Model file for the job. Use its own axes, mm. A direction names the side the tool comes from. Give positions to 0.01 mm unless a question says otherwise; leave off trailing zeros. Write each loop counter-clockwise with the first axis right and the second up, starting at its lowest first coordinate (ties: lowest second). Pieces come first, ordered by that corner, then holes. Notation, with made-up numbers: M 36,49 L 83,49 A28 cw 83,74 Z; hole C 0.5,-10.5 d2. An arc over 180 degrees is marked long. Answer as a JSON object with one key per item and string values. Group by question number.
```python
from build123d import *

# Parameters (mm, degrees)
F0_R     = 1
F0_W     = 2
F0_H     = 3
F0_R_2   = 12.5
F1_DEPTH = 2
F2_DEPTH = 2


with BuildPart() as f1:
    # F0 (on Top) → F1 (new body)
    with BuildSketch(Plane.XY):
        with BuildLine():
            Line((10, 16), (-10, 16))
            ThreePointArc((-10, 16), (-14.2426406871, 14.2426406871), (-16, 10))
            Line((-16, 10), (-16, -10))
            ThreePointArc((-16, -10), (-14.2426406871, -14.2426406871), (-10, -16))
            Line((-10, -16), (10, -16))
            ThreePointArc((10, -16), (14.2426406871, -14.2426406871), (16, -10))
            Line((16, -10), (16, 10))
            ThreePointArc((16, 10), (14.2426406871, 14.2426406871), (10, 16))
        make_face()
        with Locations((-12, -12)):
            Circle(F0_R, mode=Mode.SUBTRACT)
        with Locations((-13.5, -7.8047601065)):
            Rectangle(F0_W, F0_H, mode=Mode.SUBTRACT)
        with Locations((12, -12)):
            Circle(F0_R, mode=Mode.SUBTRACT)
        with Locations((13.5, -7.8047601065)):
            Rectangle(F0_W, F0_H, mode=Mode.SUBTRACT)
        with Locations((-13.5, 7.8047601065)):
            Rectangle(F0_W, F0_H, mode=Mode.SUBTRACT)
        with Locations((-12, 12)):
            Circle(F0_R, mode=Mode.SUBTRACT)
        Circle(F0_R_2, mode=Mode.SUBTRACT)
        with Locations((13.5, 7.8047601065)):
            Rectangle(F0_W, F0_H, mode=Mode.SUBTRACT)
        with Locations((12, 12)):
            Circle(F0_R, mode=Mode.SUBTRACT)
    extrude(amount=F1_DEPTH)

    # F0 (on Top) → F2 (join)
    with BuildSketch(Plane.XY):
        with BuildLine():
            Line((10, 16), (-10, 16))
            ThreePointArc((-10, 16), (-14.2426406871, 14.2426406871), (-16, 10))
            Line((-16, 10), (-16, -10))
            ThreePointArc((-16, -10), (-14.2426406871, -14.2426406871), (-10, -16))
            Line((-10, -16), (10, -16))
            ThreePointArc((10, -16), (14.2426406871, -14.2426406871), (16, -10))
            Line((16, -10), (16, 10))
            ThreePointArc((16, 10), (14.2426406871, 14.2426406871), (10, 16))
        make_face()
        with Locations((-12, -12)):
            Circle(F0_R, mode=Mode.SUBTRACT)
        with Locations((-13.5, -7.8047601065)):
            Rectangle(F0_W, F0_H, mode=Mode.SUBTRACT)
        with Locations((12, -12)):
            Circle(F0_R, mode=Mode.SUBTRACT)
        with Locations((13.5, -7.8047601065)):
            Rectangle(F0_W, F0_H, mode=Mode.SUBTRACT)
        with Locations((-13.5, 7.8047601065)):
            Rectangle(F0_W, F0_H, mode=Mode.SUBTRACT)
        with Locations((-12, 12)):
            Circle(F0_R, mode=Mode.SUBTRACT)
        Circle(F0_R_2, mode=Mode.SUBTRACT)
        with Locations((13.5, 7.8047601065)):
            Rectangle(F0_W, F0_H, mode=Mode.SUBTRACT)
        with Locations((12, 12)):
            Circle(F0_R, mode=Mode.SUBTRACT)
    extrude(amount=F2_DEPTH)


solid = f1.part
```
Q1. Drop flat-ended pins along their axis: P1, Ø0.6, axis at x = 13, z = 0.5, coming from the -Y side; P2, Ø0.6, axis at x = 14, z = 1, coming from the -Y side; P3, Ø1, axis at x = -14, z = 0.5, coming from the +Y side. Give the stop position or say it passes through.
Q2. Wall check: L1, parallel to X at y = 6.5, z = 0.6; L2, parallel to X at y = -8.5, z = 1.2; L3, parallel to Y at x = 8.5, z = 0.3. Give the ranges that are in metal, low to high.
Q3. Slice it at A-A, the plane x = 0. Write the cut outline in (y, z).
Q4. Slice it at B-B, the plane z = 1.45. Count the separate pieces of the cut face and the enclosed holes in it, then the cut area to 3 significant figures.
Q5. Slice it at C-C, the plane x = -12. Write the cut outline in (y, z).
Q6. 3-axis set-ups, long thin cutter, end or side, ignore diameter. For faces 1 (the flat face through (13, -6.305, 1)), 2 (the cylindrical face through (14.289, 14.196, 0.986)): which of +Z, -Z, +X, -X, +Y, -Y reach the whole face in a straight line?
Q7. Two-plate mould, pull along X, no slides. Class faces 3 (the flat face through (-14.5, -8, 1)), 4 (the flat face through (0, 16, 1)), 5 (the cylindrical face through (14.196, -14.289, 0.986)): +X half, -X half, draft (parallel to the pull), parting line (faces both ways), or undercut.
Solved:
{
 "1": {"P1": "stops at y = -15.36", "P2": "stops at y = -14.72", "P3": "stops at y = 14.87"},
 "2": {"L1": "x = -16 to -14.5, -12.5 to -10.68, 10.68 to 12.5, 14.5 to 16", "L2": "x = -16 to -14.5, -12.5 to -9.17, 9.17 to 12.5, 14.5 to 16", "L3": "y = -16 to -9.17, 9.17 to 16"},
 "3": {"outline": "M -16,0 L -12.5,0 L -12.5,2 L -16,2 Z; M 12.5,0 L 16,0 L 16,2 L 12.5,2 Z"},
 "4": {"separate pieces": "1", "enclosed holes": "9", "area": "466 mm²"},
 "5": {"outline": "M -15.66,0 L -13,0 L -13,2 L -15.66,2 Z; M -11,0 L -3.5,0 L -3.5,2 L -11,2 Z; M 3.5,0 L 11,0 L 11,2 L 3.5,2 Z; M 13,0 L 15.66,0 L 15.66,2 L 13,2 Z"},
 "6": {"face 1": "+Z, -Z", "face 2": "+Z, -Z, +X, +Y"},
 "7": {"face 3": "undercut", "face 4": "draft", "face 5": "+X half"}
}
